Verification items for the finished model (mm, model axes). Give positions to 0.01 mm unless a question says otherwise; leave off trailing zeros. Order: outer loops, then holes, each group sorted by start corner. A loop starts at its lowest first (then second) coordinate and runs counter-clockwise, first axis right, second up. Notation, with made-up numbers: (16.5, -31) -> (44.5, -31) arc R15 ccw to (44.5, -25) -> close; hole circle Ø10 at (-4.75, 75.5). An arc over 180 degrees is marked (long way). One line per question, with ' | ' between items. Start each with the question number.
Q1. Material ranges on probe 1 along Z at (x, y) = (81.5, 6); probe 2 along Z at (x, y) = (97.5, 2.5); probe 3 along Y at (x, z) = (127.5, 182), recorded low to high. Write a range as [from, to].
Q2. Section check B-B on x = 166. Record the cut outline in (y, z).
Q3. Section check A-A on y = 5.25. Record the cut outline in (x, z), plus the area to 3 significant figures.
Q4. Section check C-C on z = 400. Record the cut outline in (x, y), plus the area to 3 significant figures.
Q5. Go/stop test with flat-tipped pins: pin 1 (5 mm diameter, centred on y = 6.5, z = 495, fed in from -X); pin 2 (10 mm diameter, centred on x = 112.5, z = 361, fed in from -Y); pin 3 (3 mm diameter, centred on x = 167.5, z = 212.5, fed in from +Y). Record where each tip stops, or that it passes through.
Q6. Mould release check, pull along Z, two halves, no side actions. Record for faces 1 (the flat face through (91, 10, 178)), 2 (the conical face through (89.54, 9.61, 261.65)): released by +Z, released by -Z, zero draft, split by the parting line, or undercut.
from build123d import *

# Parameters (mm, degrees)
SKETCH1_W           = 200
SKETCH1_H           = 600
BOSS_EXTRUDE1_DEPTH = 2
SKETCH3_R           = 18
BOSS_EXTRUDE2_DEPTH = 8
BOSS_EXTRUDE2_TAPER = 40


with BuildPart() as part:
    # Sketch1 → Boss-Extrude1 (new body)
    with BuildSketch(Plane(origin=(0, 0, 0), x_dir=(1, 0, 0), z_dir=(0, 1, 0))):
        with Locations((91.05572809, -273.16718427)):
            Rectangle(SKETCH1_W, SKETCH1_H)
    extrude(amount=BOSS_EXTRUDE1_DEPTH)

    # Sketch3 → Boss-Extrude2 (add)
    with BuildSketch(Plane(origin=(0, 2, 0), x_dir=(1, 0, 0), z_dir=(0, 1, 0))):
        with Locations((91.05572809, -83.246549225)):
            Circle(SKETCH3_R)
        with Locations((91.05572809, -178.246549225)):
            Circle(SKETCH3_R)
        with Locations((91.05572809, -273.16718427)):
            Circle(SKETCH3_R)
        with Locations((91.05572809, -368.246549225)):
            Circle(SKETCH3_R)
        with Locations((91.05572809, -463.246549225)):
            Circle(SKETCH3_R)
    extrude(amount=BOSS_EXTRUDE2_DEPTH, taper=BOSS_EXTRUDE2_TAPER)


solid = part.part
Filled in:
1) probe 1: [72.15, 94.34], [167.15, 189.34], [262.07, 284.26], [357.15, 379.34], [452.15, 474.34] | probe 2: [66.89, 99.6], [161.89, 194.6], [256.81, 289.52], [351.89, 384.6], [446.89, 479.6] | probe 3: [0, 2]
2) outline: (0, -26.83) -> (2, -26.83) -> (2, 573.17) -> (0, 573.17) -> close
3) outline: circle Ø30.55 at (91.06, 83.25); circle Ø30.55 at (91.06, 178.25); circle Ø30.55 at (91.06, 273.17); circle Ø30.55 at (91.06, 368.25); circle Ø30.55 at (91.06, 463.25) | area: 3,660 mm²
4) outline: (-8.94, 0) -> (191.06, 0) -> (191.06, 2) -> (-8.94, 2) -> close | area: 400 mm²
5) pin 1: through | pin 2: y = 0 | pin 3: y = 2
6) face 1: zero draft | face 2: undercut
